from build123d import *

# Parameters (mm, degrees)
SKETCH_1_W          = 70
SKETCH_1_H          = 70
EXTRUDE_1_DEPTH     = 25
SKETCH_2_R          = 18
EXTRUDE_2_DEPTH     = 22
SKETCH_3_R          = 12.5
CUT_EXTRUDE_1_DEPTH = 6
SKETCH_5_R          = 1.5
CUT_EXTRUDE_2_DEPTH = 65.272855857
SKETCH_6_W          = 10
SKETCH_6_H          = 12
CUT_EXTRUDE_3_DEPTH = 20
SKETCH_7_R          = 3
CUT_EXTRUDE_4_DEPTH = 69.256867786
SKETCH_8_R          = 6
CUT_EXTRUDE_5_DEPTH = 8
SKETCH_9_W          = 36
SKETCH_9_H          = 36
CUT_EXTRUDE_6_DEPTH = 12
FILLET_1_R          = 2
FILLET_2_R          = 2
CHAMFER_1_SIZE      = 1
FILLET_3_R          = 1


with BuildPart() as part:
    # 草图1 → 凸台-拉伸1 (new body)
    with BuildSketch(Plane(origin=(0, 0, 0), x_dir=(1, 0, 0), z_dir=(0, 1, 0))):
        Rectangle(SKETCH_1_W, SKETCH_1_H)
    extrude(amount=EXTRUDE_1_DEPTH)

    # 草图2 → 凸台-拉伸2 (add)
    with BuildSketch(Plane(origin=(0, 25, 0), x_dir=(1, 0, 0), z_dir=(0, 1, 0))):
        with Locations(Location((0, 0, 0), (0, 0, 270))):
            Circle(SKETCH_2_R)
    extrude(amount=EXTRUDE_2_DEPTH)

    # 草图3 → 切除-拉伸1 (cut)
    with BuildSketch(Plane(origin=(0, 47, 0), x_dir=(1, 0, 0), z_dir=(0, 1, 0))):
        with Locations(Location((0, 0, 0), (0, 0, 270))):
            Circle(SKETCH_3_R)
    extrude(amount=-CUT_EXTRUDE_1_DEPTH, mode=Mode.SUBTRACT)

    # 草图5 → 切除-拉伸2 (cut, through all)
    with BuildSketch(Plane(origin=(0, 41, 0), x_dir=(1, 0, 0), z_dir=(0, 1, 0))):
        with Locations(Location((0, 10, 0), (0, 0, 270))):
            Circle(SKETCH_5_R)
        with Locations(Location((8.660254038, -5, 0), (0, 0, 270))):
            Circle(SKETCH_5_R)
        with Locations(Location((-8.660254038, -5, 0), (0, 0, 270))):
            Circle(SKETCH_5_R)
    extrude(amount=-CUT_EXTRUDE_2_DEPTH, mode=Mode.SUBTRACT)

    # 草图6 → 切除-拉伸3 (cut)
    with BuildSketch(Plane.XY):
        with Locations((0, 47)):
            Rectangle(SKETCH_6_W, SKETCH_6_H)
    extrude(amount=CUT_EXTRUDE_3_DEPTH, mode=Mode.SUBTRACT)

    # 草图7 → 切除-拉伸4 (cut, through all)
    with BuildSketch(Plane(origin=(0, 0, 0), x_dir=(1, 0, 0), z_dir=(0, 1, 0))):
        with Locations(Location((-25, 25, 0), (0, 0, 270))):
            Circle(SKETCH_7_R)
        with Locations(Location((25, 25, 0), (0, 0, 270))):
            Circle(SKETCH_7_R)
        with Locations(Location((25, -25, 0), (0, 0, 270))):
            Circle(SKETCH_7_R)
        with Locations(Location((-25, -25, 0), (0, 0, 270))):
            Circle(SKETCH_7_R)
    extrude(amount=CUT_EXTRUDE_4_DEPTH, mode=Mode.SUBTRACT)

    # 草图8 → 切除-拉伸5 (cut)
    with BuildSketch(Plane(origin=(0, 25, 0), x_dir=(1, 0, 0), z_dir=(0, 1, 0))):
        with Locations(Location((-25, 25, 0), (0, 0, 270))):
            Circle(SKETCH_8_R)
        with Locations(Location((25, 25, 0), (0, 0, 90))):
            Circle(SKETCH_8_R)
        with Locations(Location((25, -25, 0), (0, 0, 270))):
            Circle(SKETCH_8_R)
        with Locations(Location((-25, -25, 0), (0, 0, 90))):
            Circle(SKETCH_8_R)
    extrude(amount=-CUT_EXTRUDE_5_DEPTH, mode=Mode.SUBTRACT)

    # 草图9 → 切除-拉伸6 (cut)
    with BuildSketch(Plane.XZ):
        Rectangle(SKETCH_9_W, SKETCH_9_H)
    extrude(amount=-CUT_EXTRUDE_6_DEPTH, mode=Mode.SUBTRACT)

    # 圆角1
    fillet_1_edges = [part.edges().sort_by_distance(p)[0] for p in [
        (0, 25, 35),
        (18, 12, 0),
        (18, 6, 18),
        (0, 12, -18),
        (18, 6, -18),
        (-18, 12, 0),
        (-18, 6, -18),
        (0, 12, 18),
        (35, 25, 0),
        (-35, 12.5, -35),
        (35, 12.5, -35),
        (35, 12.5, 35),
        (-35, 12.5, 35),
        (0, 25, -35),
        (-35, 25, 0),
    ]]
    fillet(fillet_1_edges, radius=FILLET_1_R)

    # 圆角2
    fillet_2_edges = [part.edges().sort_by_distance(p)[0] for p in [
        (0, 25, -18),
    ]]
    fillet(fillet_2_edges, radius=FILLET_2_R)

    # 倒角1
    chamfer_1_edges = [part.edges().sort_by_distance(p)[0] for p in [
        (0, 47, -12.5),
    ]]
    chamfer(chamfer_1_edges, length=CHAMFER_1_SIZE)

    # 圆角3
    fillet_3_edges = [part.edges().sort_by_distance(p)[0] for p in [
        (-5, 47, 14.915776335),
        (5, 47, 14.915776335),
        (5, 41, 14.374027852),
        (-5, 41, 14.374027852),
    ]]
    fillet(fillet_3_edges, radius=FILLET_3_R)


solid = part.part
Can you work these out from the model? Positions are in its coordinate system, mm. A direction names the side the tool comes from. Give positions to 0.01 mm unless a question says otherwise; leave off trailing zeros. Loops run counter-clockwise (first coordinate to the right, second up) from the corner with the lowest first, then second, coordinate; pieces in that order, holes last. Notation, with made-up numbers: (29, -36) - (37, -36) arc R22 ccw to (37, 3) - close; hole circle Ø4 at (21.25, 43.25). An arc over 180 degrees is marked (long way). One line per item, written item: value.
(1) If we section it at D-D, the plane y = 4.5: List the corners of the cut face in (x, z) for me.
Verdict:
outline: (-35, -33) arc R2 ccw to (-33, -35) - (33, -35) arc R2 ccw to (35, -33) - (35, 33) arc R2 ccw to (33, 35) - (-33, 35) arc R2 ccw to (-35, 33) - close; hole circle Ø6 at (-25, -25); hole circle Ø6 at (-25, 25); hole (-18, -16) arc R2 ccw to (-16, -18) - (16, -18) arc R2 ccw to (18, -16) - (18, 16) arc R2 ccw to (16, 18) - (-18, 18) - close; hole circle Ø6 at (25, -25); hole circle Ø6 at (25, 25)
(2) If we section it at C-C, the plane z = -25: List the corners of the cut face in (x, y) for me, plus the area to 3 significant figures.
Verdict:
outline: (-35, 0) - (-28, 0) - (-28, 17) - (-31, 17) - (-31, 25) - (-33, 25) arc R2 ccw to (-35, 23) - close; (-22, 0) - (22, 0) - (22, 17) - (19, 17) - (19, 25) - (-19, 25) - (-19, 17) - (-22, 17) - close; (28, 0) - (35, 0) - (35, 23) arc R2 ccw to (33, 25) - (31, 25) - (31, 17) - (28, 17) - close
area: 1,350 mm^2
(3) I need wall thicknesses on line 1 along X through (y, z) = (21, 25); line 2 along Z through (x, y) = (25, 7); line 3 along Z through (x, y) = (25.5, 21.5). Which ranges of each line are inside material? Lowest first, please.
Verdict:
line 1: -35 to -31, -19 to 19, 31 to 35
line 2: -35 to -28, -22 to 22, 28 to 35
line 3: -35 to -30.98, -19.02 to 19.02, 30.98 to 35
(4) I'm going to push flat-ended pins straight in: pin 1 (12.5 mm diameter, centred on x = 5.5, z = 4, fed in from +Y); pin 2 (9.5 mm diameter, centred on x = -23.5, z = -27, fed in from +Y); pin 3 (2 mm diameter, centred on x = -16.5, z = -10.5, fed in from +Y); pin 4 (3 mm diameter, centred on x = 7, z = 23.5, fed in from -Y). Where does each tip first touch, or does it pass through?
Verdict:
pin 1: y = 46.55
pin 2: y = 25
pin 3: y = 25.61
pin 4: y = 0
(5) If we section it at B-B, the plane x = 0: List the corners of the cut face in (y, z) for me, plus the area to 3 significant figures.
Verdict:
outline: (0, -35) - (23, -35) arc R2 ccw to (25, -33) - (25, -20) arc R2 cw to (27, -18) - (47, -18) - (47, -13.5) - (46, -12.5) - (41, -12.5) - (41, -11.5) - (12, -11.5) - (12, -16) arc R2 cw to (10, -18) - (0, -18) - close; (0, 18) - (10, 18) arc R2 cw to (12, 16) - (12, -8.5) - (41, -8.5) - (41, 18) - (27, 18) arc R2 cw to (25, 20) - (25, 33) arc R2 ccw to (23, 35) - (0, 35) - close
area: 1,840 mm^2
(6) On a 3-axis mill with a long thin cutter (end or side, diameter ignored), from which of +Z, -Z, +X, -X, +Y, -Y can I reach the whole of each face in a straight line? I mean faces 1 (the face through (23, 0, 0)), 2 (the face through (17.43, 11.4, 0.22)), 3 (the face through (25, 21, 19)). Say none if no direction works.
Verdict:
face 1: +Z, -Z, +X, -X, -Y
face 2: -Y
face 3: +Y
(7) If we section it at A-A, the plane x = -25: List the corners of the cut face in (y, z) for me.
Verdict:
outline: (0, -35) - (23, -35) arc R2 ccw to (25, -33) - (25, -31) - (17, -31) - (17, -28) - (0, -28) - close; (0, -22) - (17, -22) - (17, -19) - (25, -19) - (25, 19) - (17, 19) - (17, 22) - (0, 22) - close; (0, 28) - (17, 28) - (17, 31) - (25, 31) - (25, 33) arc R2 ccw to (23, 35) - (0, 35) - close
(8) If we mould it in two halves opening along Z, with no side actions, what happens to faces 4 (the face through (5, 44, 14)), 5 (the face through (0.49, 43.54, -12.49)), 6 (the face through (0, 11, 35)), 7 (the face through (-25, 21, -31))? For each: released by +Z, released by -Z, zero draft, split by the parting line, or undercut.
Verdict:
face 4: zero draft
face 5: undercut
face 6: released by +Z
face 7: undercut
